Autodesk Inventor part; units mm, degrees
ref_plane "Plano inicial" through (0, 0, 0) normal (0, 0, 1) x (1, 0, 0)
ref_plane "Plano final" through (0, 0, 1000) normal (0, 0, 1) x (1, 0, 0)
ref_plane "YZ Plane" through (0, 0, 0) normal (1, 0, 0) x (0, 1, 0)
ref_plane "Plano inicial" through (0, 0, 0) normal (0, 0, 1) x (1, 0, 0)
ref_plane "Plano final" through (0, 0, 1000) normal (0, 0, 1) x (1, 0, 0)
sketch "Boceto" plane through (0, 0, 0) normal (0, 0, 1) x (1, 0, 0)
  line L0 (-9.2, 25) -> (9.2, 25)
  line L1 (15, 19.2) -> (15, -19.2)
  line L2 (9.2, -25) -> (-9.2, -25)
  line L3 (-15, -19.2) -> (-15, 19.2)
  arc A0 (-9.2, 25) -> (-15, 19.2) centre (-9.2, 19.2) ccw
  arc A1 (15, 19.2) -> (9.2, 25) centre (9.2, 19.2) ccw
  arc A2 (9.2, -25) -> (15, -19.2) centre (9.2, -19.2) ccw
  arc A3 (-15, -19.2) -> (-9.2, -25) centre (-9.2, -19.2) ccw
  line L4 (-22.6817, 0) -> (22.6817, 0) construction
  line L5 (0, -36.6817) -> (0, 36.6817) construction
  arc A4 (-9.2, 22.1) -> (-12.1, 19.2) centre (-9.2, 19.2) ccw
  line L6 (-9.2, 22.1) -> (9.2, 22.1)
  arc A5 (12.1, 19.2) -> (9.2, 22.1) centre (9.2, 19.2) ccw
  line L7 (12.1, 19.2) -> (12.1, -19.2)
  arc A6 (9.2, -22.1) -> (12.1, -19.2) centre (9.2, -19.2) ccw
  line L8 (9.2, -22.1) -> (-9.2, -22.1)
  arc A7 (-12.1, -19.2) -> (-9.2, -22.1) centre (-9.2, -19.2) ccw
  line L9 (-12.1, -19.2) -> (-12.1, 19.2)
  point P0 (-15, 25)
  point P1 (15, -25)
  point P2 (15, 25)
  dimension "b" = 30
  dimension "ParH" = 50
  dimension "msp_r" = 5.8
  dimension "d8" = 15
  dimension "d9" = 25
  dimension "d10" = 2.9
extrude "Cuerpo" add sketch "Boceto" along normal up to surface (1000 mm away) from surface at 0
sketch "Sketch2" plane through (0, 0, 0) normal (0, 0, 1) x (1, 0, 0)
  line L0 (0, 0) -> (10, 0)
ref_plane "Work Plane3" through (0, 0, 0) normal (0, -1, 0) x (1, 0, 0)
sketch "Sketch3" plane through (0, 0, 0) normal (0, -1, 0) x (1, 0, 0)
  line L0 (-2, 0) -> (12, 0)
  line L1 (-2, 1000) -> (12, 1000)
  dimension "d14" = 1000
equation "\"msp_r\" = 2 * ParT"
equation "\"d8\" = 0.5 * b"
equation "\"d9\" = 0.5 * ParH"
equation "\"d10\" = ParT"
equation "\"G_OFFSET_START\" = 0"
equation "\"G_OFFSET_END\" = 0"
equation "\"G_L\" = d14"
properties part number "DIN 59 410 - 50x30x2.9-1000" material "Acero, suave"
Geometry check sheet. Reference: the model listing, model coordinates, mm. A direction names the side the tool comes from. Coordinates: 2 decimals unless noted, no trailing zeros. Order: outer loops, then holes, each group sorted by start corner. A loop starts at its lowest first (then second) coordinate and runs counter-clockwise, first axis right, second up. Notation, with made-up numbers: (68, 86) - (110, 86) arc R26 cw to (110, 111) - close; hole circle Ø3 at (46, 39). An arc over 180 degrees is marked (long way). Answer in a Markdown table with one row per item. Add a question column.
1. Section check C-C (x = 0.5). Enter the section's corners in (y, z), plus the area to 3 significant figures.
2. Section check A-A (y = 4). Enter the section's corners in (x, z), plus the area to 3 significant figures.
3. Material ranges on L1, parallel to Y at x = -2.25, z = 457.5; L2, parallel to X at y = 0, z = 904.5; L3, parallel to X at y = 20, z = 932, recorded low to high. Write a range as [from, to].
4. Access from +Z, -Z, +X, -X, +Y, -Y to the whole of each face (thin tool, end or side, straight path). Record for faces 5 (the face through (-12.3, 2, 1000)), 6 (the face through (0, -22.1, 493)).
5. Draft check along Y on faces 1 (the face through (0, 25, 493)), 2 (the face through (-12.1, 0, 493)), 3 (the face through (0, -25, 493)), 4 (the face through (15, 0, 493)). Enter one of: +Y half, -Y half, draft (parallel to the pull), parting line (faces both ways), or undercut.
6. Section check B-B (z = 207.5). Enter the section's corners in (x, y), plus the area to 3 significant figures.
Data:
| question | item | result |
|---|---|---|
| 1 | outline | (-25, 0) - (-22.1, 0) - (-22.1, 1000) - (-25, 1000) - close; (22.1, 0) - (25, 0) - (25, 1000) - (22.1, 1000) - close |
| 1 | area | 5,800 mm² |
| 2 | outline | (-15, 0) - (-12.1, 0) - (-12.1, 1000) - (-15, 1000) - close; (12.1, 0) - (15, 0) - (15, 1000) - (12.1, 1000) - close |
| 2 | area | 5,800 mm² |
| 3 | L1 | y = [-25, -22.1], [22.1, 25] |
| 3 | L2 | x = [-15, -12.1], [12.1, 15] |
| 3 | L3 | x = [-14.94, -11.99], [11.99, 14.94] |
| 4 | face 5 | +Z, +X, -X, +Y, -Y |
| 4 | face 6 | +Z, -Z |
| 5 | face 1 | +Y half |
| 5 | face 2 | undercut |
| 5 | face 3 | -Y half |
| 5 | face 4 | draft |
| 6 | outline | (-15, -19.2) arc R5.8 ccw to (-9.2, -25) - (9.2, -25) arc R5.8 ccw to (15, -19.2) - (15, 19.2) arc R5.8 ccw to (9.2, 25) - (-9.2, 25) arc R5.8 ccw to (-15, 19.2) - close; hole (-12.1, -19.2) arc R2.9 ccw to (-9.2, -22.1) - (9.2, -22.1) arc R2.9 ccw to (12.1, -19.2) - (12.1, 19.2) arc R2.9 ccw to (9.2, 22.1) - (-9.2, 22.1) arc R2.9 ccw to (-12.1, 19.2) - close |
| 6 | area | 409 mm² |
